The model under review builds one solid part; all positions refer to its coordinate system, in mm. Face numbers are marked on the shaded views. A direction names the side the tool comes from. Coordinates: 2 decimals unless noted, no trailing zeros. Order: outer loops, then holes, each group sorted by start corner. A loop starts at its lowest first (then second) coordinate and runs counter-clockwise, first axis right, second up.
```python
from build123d import *

# Parameters (mm, degrees)
F1_DEPTH = 25.4
F2_DEPTH = 25.4
F4_DEPTH = 50.8
F6_DEPTH = 50.8


# Not quite as in the source:
# - a feature names something its author has since deleted; it is built from what else it names


with BuildPart() as f1:
    # F0 (on Front) → F1 (new body)
    with BuildSketch(Plane.XZ):
        Polygon((-24.6924351323, 51.1944131529), (-62.7924351323, 51.1944131529), (-62.7924351323, 19.4444131529), (-50.0924351323, 19.4444131529), (-50.0924351323, 25.7944131529), (-37.3924351323, 25.7944131529), (-37.3924351323, 19.4444131529), (-24.6924351323, 19.4444131529), align=None)
    extrude(amount=F1_DEPTH)

    # F0 (on Front) + F1_face (on face) → F2 (join)
    with BuildSketch(Plane.XZ):
        Polygon((-24.6924351323, 51.1944131529), (-62.7924351323, 51.1944131529), (-62.7924351323, 19.4444131529), (-50.0924351323, 19.4444131529), (-50.0924351323, 25.7944131529), (-37.3924351323, 25.7944131529), (-37.3924351323, 19.4444131529), (-24.6924351323, 19.4444131529), align=None)
    with BuildSketch(Plane(origin=(-43.7424351323, -25.4, 36.2265560101), x_dir=(1, 0, 0), z_dir=(0, -1, 0))):
        Polygon((19.05, 14.9678571429), (-19.05, 14.9678571429), (-19.05, -16.7821428571), (-6.35, -16.7821428571), (-6.35, -10.4321428571), (6.35, -10.4321428571), (6.35, -16.7821428571), (19.05, -16.7821428571), align=None)
    extrude(amount=F2_DEPTH)

    # F3 (on face) → F4 (cut)
    with BuildSketch(Plane.XZ.offset(50.8)):
        Polygon((-62.7924351323, 19.4444131529), (-50.0924351323, 51.1944131529), (-62.7924351323, 51.1944131529), align=None)
    extrude(amount=-F4_DEPTH, mode=Mode.SUBTRACT)

    # F5 (on face) → F6 (cut)
    with BuildSketch(Plane.XZ.offset(50.8)):
        Polygon((-24.6924351323, 51.1944131529), (-37.3924351323, 51.1944131529), (-24.6924351323, 19.4444131529), align=None)
    extrude(amount=-F6_DEPTH, mode=Mode.SUBTRACT)


solid = f1.part
```
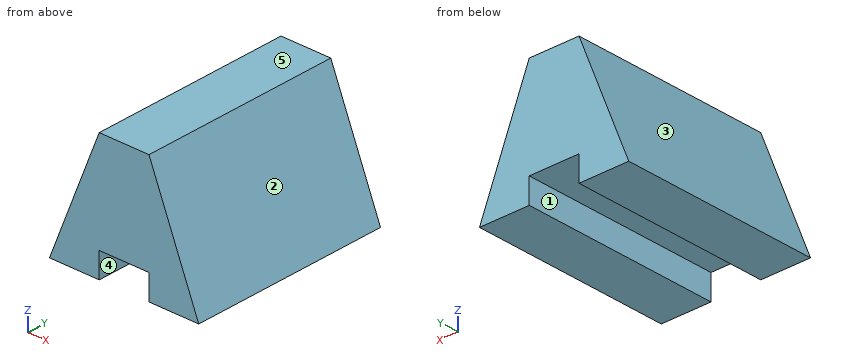
(1) We need section B-B, the plane x = -46. Write out the cut boundary in (y, z), and give its area (3 significant figures).
A:
outline: (-50.8, 25.79) - (0, 25.79) - (0, 51.19) - (-50.8, 51.19) - close
area: 1,290 mm2
(2) We need section C-C, the plane z = 29. Write out the cut boundary in (x, y).
A:
outline: (-58.97, -50.8) - (-28.51, -50.8) - (-28.51, 0) - (-58.97, 0) - close
(3) Wall thickness on probe 1 along X at (y, z) = (-33, 23); probe 2 along Z at (x, y) = (-39, -44); probe 3 along X at (y, z) = (-40.5, 25): over which ranges is each line inside the solid? List them lowest first.
A:
probe 1: x = -61.37 to -50.09, -37.39 to -26.11
probe 2: z = 25.79 to 51.19
probe 3: x = -60.57 to -50.09, -37.39 to -26.91
(4) Machinability: for the marked faces 1 and 2, which of the approach directions +Z, -Z, +X, -X, +Y, -Y give a long, thin tool a straight path to every point of the face, cutting with its end or side? Answer none if there is none.
A:
face 1: -Z, +Y, -Y
face 2: +Z, +X, +Y, -Y
(5) We need section A-A, the plane y = -44. Write out the cut boundary in (x, z).
A:
outline: (-62.79, 19.44) - (-50.09, 19.44) - (-50.09, 25.79) - (-37.39, 25.79) - (-37.39, 19.44) - (-24.69, 19.44) - (-37.39, 51.19) - (-50.09, 51.19) - close
(6) Draft analysis for pull direction X (two halves, no side actions). For the marked faces 3, 4 and 5, state which applies: released by +X, released by -X, zero draft, split by the parting line, or undercut.
A:
face 3: released by -X
face 4: undercut
face 5: zero draft
(7) For pin 1 Ø1 at (y, z) = (-13, 36.5) entering from -X; pin 2 Ø3 at (y, z) = (-17, 23.5) entering from +X; pin 3 Ø6.5 at (x, y) = (-45, -29.5) entering from -Z; pin 4 Ø1.5 at (x, z) = (-33.5, 44) entering from -Y, all flat-tipped, find the tip position at first contact; note any pin that passes through.
A:
pin 1: stops at x = -56.17
pin 2: stops at x = -25.71
pin 3: stops at z = 25.79
pin 4: passes through
